The model under review builds one solid part; all positions refer to its coordinate system, in mm. A direction names the side the tool comes from. Round coordinates to 2 decimals unless told otherwise and drop trailing zeros. Write each loop counter-clockwise with the first axis right and the second up, starting at its lowest first coordinate (ties: lowest second). Pieces come first, ordered by that corner, then holes. Notation, with made-up numbers: M 88,8.5 L 128,8.5 A26 cw 128,30.5 Z; hole C 69,-10 d2. An arc over 180 degrees is marked long. Write item = value, one per line. Start each with the question number.
Item 1: Take a section at D-D, the plane x = 15. Give the boundary of the cut face in (y, z).
Item 2: The part is to be moulded in two halves that separate along Z. For faces 1 (the flat face through (15, -6, 0)), 2 (the cylindrical face through (4.77, -4.44, -5.72)), 3 (the flat face through (15, 0, -11)), say which applies: +Z half, -Z half, draft (parallel to the pull), parting line (faces both ways), or undercut.
Item 3: Take a section at B-B, the plane z = -4.5. Give the boundary of the cut face in (x, y), plus the area to 3 significant figures.
Item 4: To check wall thickness, follow line 1 along Z through (x, y) = (25.5, -10.6); line 2 along X through (y, z) = (-7, -4.5); line 3 along Z through (x, y) = (21.5, -7.5). State the ranges of each line that lie inside material, in increasing order.
Item 5: Take a section at C-C, the plane y = -9.75. Give the boundary of the cut face in (x, z), plus the area to 3 significant figures.
Item 6: Take a section at A-A, the plane x = 25.5. Give the boundary of the cut face in (y, z).
Item 7: Tool access review of faces 4 (the cylindrical face through (12.905, -1.479, -21.747)), 5 (the flat face through (27, -9, -4)), 6 (the cylindrical face through (24.345, -4.437, -25.979)): name each direction out of +Z, -Z, +X, -X, +Y, -Y from which nothing blocks a thin tool from reaching the whole face with its end or side.
Item 8: For pin 1 Ø1.8 at (x, z) = (9, -14) entering from +Y; pin 2 Ø3 at (x, z) = (25.5, -26) entering from -Y; pin 3 Ø4 at (x, z) = (21.46, -15) entering from -Y, all flat-tipped, find the tip position at first contact; note any pin that passes through.
from build123d import *

# Parameters (mm, degrees)
F0_W      = 30
F0_H      = 30
F0_R      = 10
F0_R_2    = 3
F1_DEPTH  = 12
F2_R      = 1.25
F3_DEPTH  = 20
F4_DEPTH  = 3
F5_R      = 3
F5_R_2    = 1.25
F6_DEPTH  = 3
F8_DEPTH  = 3
F9_DEPTH  = 3
F12_D     = 3
F14_D     = 4.2
F14_DEPTH = 5
F14_TIP   = 1.2618073
F15_SIZE  = 0.25


# Not quite as in the source:
# - a feature names something its author has since deleted; it is built from what else it names


with BuildPart() as f1:
    # F0 (on Front) → F1 (new body)
    with BuildSketch(Plane.XZ):
        with Locations((15, -15)):
            Rectangle(F0_W, F0_H)
        with Locations((15, -15)):
            Circle(F0_R, mode=Mode.SUBTRACT)
        with Locations((15, -15)):
            Circle(F0_R)
        with Locations((15, -16.066)):
            Circle(F0_R_2, mode=Mode.SUBTRACT)
        with Locations((15, -16.066)):
            Circle(F0_R_2)
    extrude(amount=F1_DEPTH)

    # F2 (on face) → F3 (cut)
    with BuildSketch(Plane(origin=(0, 0, 0), x_dir=(-1, 0, 0), z_dir=(0, 1, 0))):
        with Locations((-4.5, -4.5)):
            Circle(F2_R)
        with Locations((-25.5, -4.5)):
            Circle(F2_R)
        with Locations((-25.5, -25.5)):
            Circle(F2_R)
        with Locations((-4.5, -25.5)):
            Circle(F2_R)
    extrude(amount=-F3_DEPTH, mode=Mode.SUBTRACT)

    # F0 (on Front) → F4 (cut)
    with BuildSketch(Plane.XZ):
        with Locations((15, -16.066)):
            Circle(F0_R_2)
    extrude(amount=F4_DEPTH, mode=Mode.SUBTRACT)

    # F5 (on face) → F6 (cut)
    with BuildSketch(Plane.XZ.offset(12)):
        with Locations((4.5, -4.5)):
            Circle(F5_R)
        with Locations((4.5, -4.5)):
            Circle(F5_R_2, mode=Mode.SUBTRACT)
        with Locations((25.5, -4.5)):
            Circle(F5_R)
        with Locations((25.5, -4.5)):
            Circle(F5_R_2, mode=Mode.SUBTRACT)
        with Locations((4.5, -25.5)):
            Circle(F5_R)
        with Locations((4.5, -25.5)):
            Circle(F5_R_2, mode=Mode.SUBTRACT)
        with Locations((25.5, -25.5)):
            Circle(F5_R)
        with Locations((25.5, -25.5)):
            Circle(F5_R_2, mode=Mode.SUBTRACT)
    extrude(amount=-F6_DEPTH, mode=Mode.SUBTRACT)

    # F7 (on face) → F8 (cut)
    with BuildSketch(Plane(origin=(0, 0, 0), x_dir=(-1, 0, 0), z_dir=(0, 1, 0))):
        with BuildLine():
            Line((-17.9580398915, -15.566), (-19.9749371855, -15.566))
            ThreePointArc((-19.9749371855, -15.566), (-20, -16.066), (-19.9749371855, -16.566))
            Line((-19.9749371855, -16.566), (-17.9580398915, -16.566))
            ThreePointArc((-17.9580398915, -16.566), (-18, -16.066), (-17.9580398915, -15.566))
        make_face()
    extrude(amount=-F8_DEPTH, mode=Mode.SUBTRACT)

    # F7 (on face) → F9 (cut)
    with BuildSketch(Plane(origin=(0, 0, 0), x_dir=(-1, 0, 0), z_dir=(0, 1, 0))):
        with BuildLine():
            ThreePointArc((-18.4208497185, -12.4193868859), (-18.4150519192, -9.7016030586), (-21.128355545, -9.8576991225))
            ThreePointArc((-21.128355545, -9.8576991225), (-22.8195543866, -16.6895470386), (-18.4586259046, -22.2137304394))
            ThreePointArc((-18.4586259046, -22.2137304394), (-17.1046358453, -21.7662439553), (-17.5, -20.3961270189))
            ThreePointArc((-17.5, -20.3961270189), (-19.1995404186, -18.7796433577), (-19.9749371855, -16.566))
            Line((-19.9749371855, -16.566), (-21.5030275285, -16.566))
            ThreePointArc((-21.5030275285, -16.566), (-22.0030275285, -16.066), (-21.5030275285, -15.566))
            Line((-21.5030275285, -15.566), (-19.9749371855, -15.566))
            ThreePointArc((-19.9749371855, -15.566), (-19.4830350162, -13.8518642672), (-18.4208497185, -12.4193868859))
        make_face()
        with BuildLine():
            ThreePointArc((-11.5413740954, -22.2137304394), (-7.1804456134, -16.6895470386), (-8.871644455, -9.8576991225))
            ThreePointArc((-8.871644455, -9.8576991225), (-11.5849480808, -9.7016030586), (-11.5791502815, -12.4193868859))
            ThreePointArc((-11.5791502815, -12.4193868859), (-10.0329877054, -16.6394011384), (-12.5, -20.3961270189))
            ThreePointArc((-12.5, -20.3961270189), (-12.8953641547, -21.7662439553), (-11.5413740954, -22.2137304394))
        make_face()
        with BuildLine():
            ThreePointArc((-19.9749371855, -16.566), (-20, -16.066), (-19.9749371855, -15.566))
            Line((-19.9749371855, -15.566), (-21.5030275285, -15.566))
            ThreePointArc((-21.5030275285, -15.566), (-22.0030275285, -16.066), (-21.5030275285, -16.566))
            Line((-21.5030275285, -16.566), (-19.9749371855, -16.566))
        make_face()
    extrude(amount=-F9_DEPTH, mode=Mode.SUBTRACT)

    # F12 (through all)
    with Locations(Plane(origin=(0, 0, 0), x_dir=(-1, 0, 0), z_dir=(0, 1, 0))):
        with Locations((-21.456294, -15), (-8.543706, -15)):
            Hole(F12_D / 2)

    # F14
    with Locations(Plane.XZ.offset(12)):
        with Locations((8.543706, -15), (21.456294, -15)):
            Hole(F14_D / 2, depth=F14_DEPTH)
            with Locations((0, 0, -(F14_DEPTH + F14_TIP / 2))):  # 118° drill point
                Cone(0, F14_D / 2, F14_TIP, mode=Mode.SUBTRACT)

    # F15
    f15_edges = [f1.edges().sort_by_distance(p)[0] for p in [
        (15, -12, 0),
        (30, -12, -15),
        (0, -12, -15),
        (15, -12, -30),
        (1.5, -12, -25.5),
        (22.5, -12, -25.5),
        (6.443706, -12, -15),
        (1.5, -12, -4.5),
        (19.356294, -12, -15),
        (22.5, -12, -4.5),
        (0, -6, 0),
        (30, -6, 0),
        (30, -6, -30),
        (0, -6, -30),
    ]]
    chamfer(f15_edges, length=F15_SIZE)


solid = f1.part
Response values:
q1.outline = M -12,-29.75 L -11.75,-30 L 0,-30 L 0,-19.07 L -3,-19.07 L -3,-13.07 L 0,-13.07 L 0,0 L -11.75,0 L -12,-0.25 Z
q2.face_1 = +Z half
q2.face_2 = undercut
q2.face_3 = draft
q3.outline = M 0,-11.75 L 0.25,-12 L 1.25,-12 L 1.5,-11.75 L 1.5,-9 L 3.25,-9 L 3.25,0 L 0,0 Z; M 5.75,-9 L 7.5,-9 L 7.5,-11.75 L 7.75,-12 L 22.25,-12 L 22.5,-11.75 L 22.5,-9 L 24.25,-9 L 24.25,0 L 5.75,0 Z; M 26.75,-9 L 28.5,-9 L 28.5,-11.75 L 28.75,-12 L 29.75,-12 L 30,-11.75 L 30,0 L 26.75,0 Z
q3.area = 279 mm2
q4.line_1 = -30 to -28.5, -22.5 to -7.5, -1.5 to 0
q4.line_2 = 0 to 3.25, 5.75 to 24.25, 26.75 to 30
q4.line_3 = -30 to -17.1, -12.9 to 0
q5.outline = M 0,-29.75 L 0.25,-30 L 29.75,-30 L 30,-29.75 L 30,-0.25 L 29.75,0 L 0.25,0 L 0,-0.25 Z; hole C 4.5,-25.5 d6; hole C 4.5,-4.5 d6; hole C 8.54,-15 d4.2; hole C 21.46,-15 d4.2; hole C 25.5,-25.5 d6; hole C 25.5,-4.5 d6
q5.area = 759 mm2
q6.outline = M -12,-29.75 L -11.75,-30 L 0,-30 L 0,-26.75 L -9,-26.75 L -9,-28.5 L -11.75,-28.5 L -12,-28.75 Z; M -12,-22.25 L -11.75,-22.5 L -9,-22.5 L -9,-24.25 L 0,-24.25 L 0,-5.75 L -9,-5.75 L -9,-7.5 L -11.75,-7.5 L -12,-7.75 Z; M -12,-1.25 L -11.75,-1.5 L -9,-1.5 L -9,-3.25 L 0,-3.25 L 0,0 L -11.75,0 L -12,-0.25 Z
q7.face_4 = +Y
q7.face_5 = -Y
q7.face_6 = +Y, -Y
q8.pin_1 = -3
q8.pin_2 = -9
q8.pin_3 = -6.94
